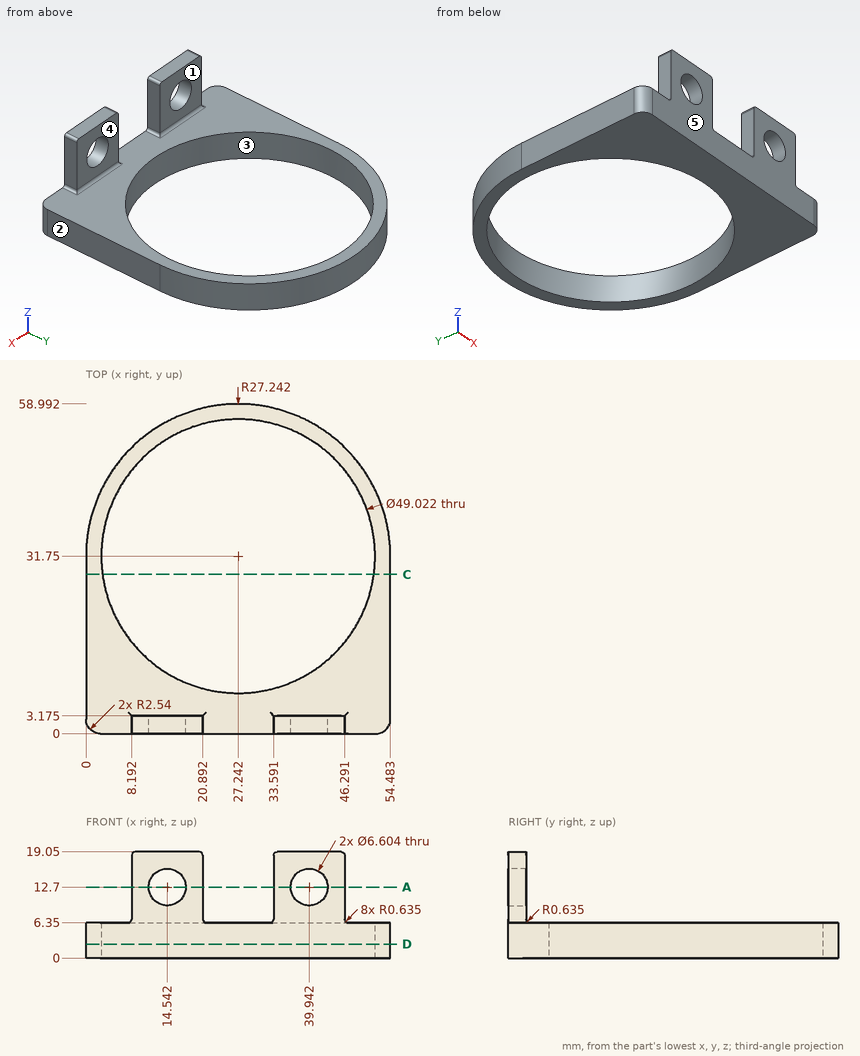
Design review of the part shown in the three views and the two pictorial views. Dimensions are in mm from the part's minimum x, y and z. A direction names the side the tool comes from. Round coordinates to 2 decimals unless told otherwise and drop trailing zeros. Write each loop counter-clockwise with the first axis right and the second up, starting at its lowest first coordinate (ties: lowest second). Pieces come first, ordered by that corner, then holes. Notation, with made-up numbers: M 5,23 L 28,23 A21 ccw 28,60 Z; hole C 88,51 d1. An arc over 180 degrees is marked long. One line per item, written item: value. Start each with the question number.
1. Take a section at D-D on z = 2.5. State the section outline as (x, y) points.
2. For the marked faces 4 and 5, list the 3-axis set-ups (+Z, -Z, +X, -X, +Y, -Y) from which the entire face can be reached by the end or side of a thin tool; tool diameter is ignored.
3. Take a section at A-A on z = 12.7. State the section outline as (x, y) points (1 decimal).
4. Clearance check with flat-ended pins moving along their axes: P1, Ø2.5, axis at y = 2, z = 10.5, coming from the -X side; P2, Ø3.5, axis at y = 1.5, z = 15, coming from the +X side; P3, Ø5, axis at x = 47, z = 4, coming from the +Y side. State where each tip first meets the part, or that it passes through.
5. Take a section at C-C on y = 28.5. State the section outline as (x, z) points.
6. Draft analysis for pull direction Y (two halves, no side actions). For the marked faces 1, 2 and 3, state which applies: pulls with the +Y half, pulls with the -Y half, needs draft (parallel to the pull), parting line crosses it, or undercut.
7. To check wall thickness, follow probe 1 along X at (y, z) = (0.75, 12.7); probe 2 along Y at (x, z) = (41.5, 15.75) (1 decimal); probe 3 along X at (y, z) = (27, 2.75) (1 decimal). State the ranges of each line that lie inside material, in increasing order. Write a range as from..to.
Computed:
1. outline: M 0,2.54 A2.54 ccw 2.54,0 L 51.94,0 A2.54 ccw 54.48,2.54 L 54.48,31.75 A27.24 ccw 0,31.75 Z; hole C 27.24,31.75 d49.02
2. face 4: +Z, +X, -X, +Y
2. face 5: +Z, -Z, +X, -X, -Y
3. outline: M 8.2,0 L 11.2,0 L 11.2,3.2 L 8.2,3.2 Z; M 17.8,0 L 20.9,0 L 20.9,3.2 L 17.8,3.2 Z; M 33.6,0 L 36.6,0 L 36.6,3.2 L 33.6,3.2 Z; M 43.2,0 L 46.3,0 L 46.3,3.2 L 43.2,3.2 Z
4. P1: stops at x = 8.19
4. P2: stops at x = 46.29
4. P3: stops at y = 52.83
5. outline: M 0,0 L 2.95,0 L 2.95,6.35 L 0,6.35 Z; M 51.54,0 L 54.48,0 L 54.48,6.35 L 51.54,6.35 Z
6. face 1: pulls with the +Y half
6. face 2: needs draft
6. face 3: undercut
7. probe 1: x = 8.19..11.24, 17.84..20.89, 33.59..36.64, 43.24..46.29
7. probe 2: y = 0..3.2
7. probe 3: x = 0..3.2, 51.3..54.5
